Could you check a few things on this model? Use its own coordinates, in mm. Round coordinates to 2 decimals unless told otherwise and drop trailing zeros. Order: outer loops, then holes, each group sorted by start corner. A loop starts at its lowest first (then second) coordinate and runs counter-clockwise, first axis right, second up. Notation, with made-up numbers: M 3.5,-28.75 L 23.5,-28.75 A22 ccw 23.5,10.25 Z; hole C 43,-22 d6. An arc over 180 degrees is marked long. Write each question's results on one line, items separated by ' | '. Start each with the question number.
1. Please list where these lines run through material, in increasing order: L1, parallel to Y at x = -115.5, z = -0.55; L2, parallel to Y at x = -35.5, z = 0.65; L3, parallel to X at y = -23, z = 0.8.
2. I'm going to push flat-ended pins straight in: pin 1 (0.8 mm diameter, centred on x = -42, z = -0.5, fed in from +Y); pin 2 (1 mm diameter, centred on x = -39.5, z = -1, fed in from -Y); pin 3 (1.1 mm diameter, centred on x = -37, z = 0.5, fed in from +Y). Where does each tip first touch, or does it pass through?
3. Suppose I cut it at A-A on z = 0.4. Write out the boundary of the cut face in (x, y).
4. Suppose I cut it at B-B on y = -19. Write out the boundary of the cut face in (x, z).
5. Suppose I cut it at C-C on x = -108.5. Write out the boundary of the cut face in (y, z), and give its area (3 significant figures).
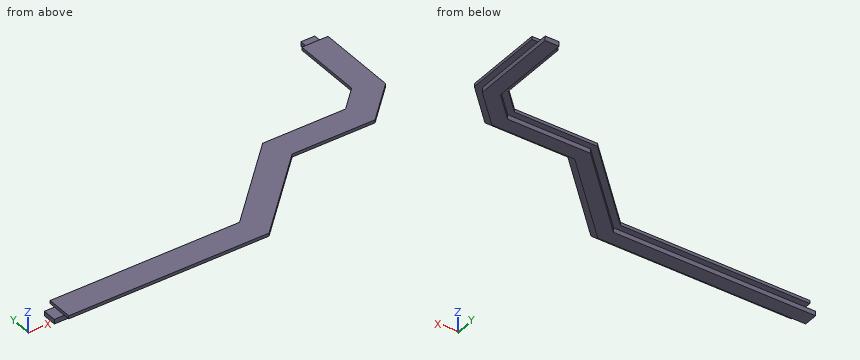
Autodesk Inventor part; units mm, degrees
ref_plane "YZ Plane" through (0, 0, 0) normal (1, 0, 0) x (0, 1, 0)
ref_plane "XZ Plane" through (0, 0, 0) normal (0, 1, 0) x (-1, 0, 0)
ref_plane "XY Plane" through (0, 0, 0) normal (0, 0, 1) x (1, 0, 0)
sketch "Эскиз1" plane through (0, 0, 0) normal (0, 0, 1) x (1, 0, 0)
  line L0 (-75.0711, -58) -> (-141.1512, -58)
  line L1 (-141.1512, -58) -> (-141.1512, -4.9289)
  line L2 (-141.1512, -4.9289) -> (-133.2223, 3)
  line L3 (-14, 3) -> (-133.2223, 3)
  line L4 (-14, 3) -> (-14, -24.0711)
  line L5 (-14, -24.0711) -> (-21.9289, -32)
  line L6 (-21.9289, -32) -> (-49.0711, -32)
  line L7 (-49.0711, -32) -> (-75.0711, -58)
  line L8 (-131.1512, -2) -> (-136.1512, -7)
  line L9 (-136.1512, -7) -> (-136.1512, -13.8712)
  line L10 (-136.1512, -13.8712) -> (-136.1512, -19.5281)
  line L11 (-136.1512, -19.5281) -> (-136.1512, -26.3992)
  line L12 (-136.1512, -26.3992) -> (-136.1512, -27)
  line L13 (-136.1512, -27) -> (-131.0951, -27)
  line L14 (-131.0951, -27) -> (-124.224, -27)
  line L15 (-124.224, -27) -> (-118.5671, -27)
  line L16 (-118.5671, -27) -> (-111.696, -27)
  line L17 (-111.696, -27) -> (-106.0391, -27)
  line L18 (-106.0391, -27) -> (-99.168, -27)
  line L19 (-99.168, -27) -> (-93.5111, -27)
  line L20 (-93.5111, -27) -> (-86.64, -27)
  line L21 (-86.64, -27) -> (-80.9831, -27)
  line L22 (-80.9831, -27) -> (-74.112, -27)
  line L23 (-74.112, -27) -> (-68.4551, -27)
  line L24 (-68.4551, -27) -> (-61.584, -27)
  line L25 (-61.584, -27) -> (-55.9271, -27)
  line L26 (-55.9271, -27) -> (-49.056, -27)
  line L27 (-49.056, -27) -> (-43.3991, -27)
  line L28 (-43.3991, -27) -> (-36.528, -27)
  line L29 (-36.528, -27) -> (-30.8711, -27)
  line L30 (-30.8711, -27) -> (-24, -27)
  line L31 (-24, -27) -> (-19, -22)
  line L32 (-19, -22) -> (-19, -15.1289)
  line L33 (-19, -15.1289) -> (-19, -9.472)
  line L34 (-19, -9.472) -> (-19, -2.6009)
  line L35 (-19, -2.6009) -> (-19, -2)
  line L36 (-19, -2) -> (-24.056, -2)
  line L37 (-24.056, -2) -> (-30.9271, -2)
  line L38 (-30.9271, -2) -> (-36.584, -2)
  line L39 (-36.584, -2) -> (-43.4551, -2)
  line L40 (-43.4551, -2) -> (-49.112, -2)
  line L41 (-49.112, -2) -> (-55.9831, -2)
  line L42 (-55.9831, -2) -> (-61.64, -2)
  line L43 (-61.64, -2) -> (-68.5111, -2)
  line L44 (-68.5111, -2) -> (-74.168, -2)
  line L45 (-74.168, -2) -> (-81.0391, -2)
  line L46 (-81.0391, -2) -> (-86.696, -2)
  line L47 (-86.696, -2) -> (-93.5671, -2)
  line L48 (-93.5671, -2) -> (-99.224, -2)
  line L49 (-99.224, -2) -> (-106.0951, -2)
  line L50 (-106.0951, -2) -> (-111.752, -2)
  line L51 (-111.752, -2) -> (-118.6231, -2)
  line L52 (-118.6231, -2) -> (-124.28, -2)
  line L53 (-124.28, -2) -> (-131.1512, -2)
  line L54 (-141.1512, -69.9) -> (-42.8584, -69.9)
  line L55 (-141.1512, -63) -> (-141.1512, -69.9)
  line L56 (-141.1512, -63) -> (-73, -63)
  line L57 (-73, -63) -> (-47, -37)
  line L58 (-47, -37) -> (-19.8579, -37)
  line L59 (-19.8579, -37) -> (-9, -26.1421)
  line L60 (-9, -26.1421) -> (-9, 3)
  line L61 (-9, 3) -> (-2, 3)
  line L62 (-2, -29.0416) -> (-2, 3)
  line L63 (-42.8584, -69.9) -> (-2, -29.0416)
  line L64 (-73.0828, -62.8) -> (-141.3512, -62.8)
  line L65 (-141.3512, -62.8) -> (-141.3512, -70.1)
  line L66 (-141.3512, -70.1) -> (-42.7755, -70.1)
  line L67 (-42.7755, -70.1) -> (-1.8, -29.1245)
  line L68 (-1.8, -29.1245) -> (-1.8, 3.2)
  line L69 (-1.8, 3.2) -> (-9.2, 3.2)
  line L70 (-9.2, 3.2) -> (-9.2, -26.0593)
  line L71 (-9.2, -26.0593) -> (-19.9407, -36.8)
  line L72 (-19.9407, -36.8) -> (-47.0828, -36.8)
  line L73 (-47.0828, -36.8) -> (-73.0828, -62.8)
  line L74 (-141.3512, -58.2) -> (-74.9882, -58.2)
  line L75 (-74.9882, -58.2) -> (-48.9882, -32.2)
  line L76 (-48.9882, -32.2) -> (-21.8461, -32.2)
  line L77 (-21.8461, -32.2) -> (-13.8, -24.1539)
  line L78 (-13.8, -24.1539) -> (-13.8, 3.2)
  line L79 (-13.8, 3.2) -> (-133.3051, 3.2)
  line L80 (-133.3051, 3.2) -> (-141.3512, -4.8461)
  line L81 (-141.3512, -4.8461) -> (-141.3512, -58.2)
  line L82 (-141.1512, -58) -> (-141.1512, -66.7)
  line L83 (-5.3, 3) -> (-14, 3)
  line L84 (-44.9289, -42) -> (-65.9289, -63)
  line L85 (-65.9289, -63) -> (-45.8579, -63)
  line L86 (-45.8579, -63) -> (-24.8579, -42)
  line L87 (-24.8579, -42) -> (-44.9289, -42)
  point P0 (-9.2, 3)
  point P1 (-13.8, 3)
  point P2 (-141.1512, -58.2)
  point P3 (-141.1512, -62.8)
  dimension "d10" = 0.2
  dimension "d11" = 0.2
extrude "Выдавливание1" add sketch "Эскиз1" against normal blind 1.5 contours L74 L75 L76 L77 L78 L83 L70 L71 L72 L73 L64 L82
sketch "Эскиз2" plane through (0, 0, 0) normal (0, 0, 1) x (1, 0, 0)
  line L0 (-19.9407, -36.8) -> (-47.0828, -36.8)
  line L1 (-47.0828, -36.8) -> (-73.0828, -62.8)
  line L2 (-73.0828, -62.8) -> (-141.1512, -62.8)
  line L3 (-141.1512, -62.8) -> (-141.1512, -58.2)
  line L4 (-141.1512, -58.2) -> (-74.9882, -58.2)
  line L5 (-74.9882, -58.2) -> (-48.9882, -32.2)
  line L6 (-48.9882, -32.2) -> (-21.8461, -32.2)
  line L7 (-21.8461, -32.2) -> (-13.8, -24.1539)
  line L8 (-13.8, -24.1539) -> (-13.8, 3)
  line L9 (-13.8, 3) -> (-9.2, 3)
  line L10 (-9.2, 3) -> (-9.2, -26.0593)
  line L11 (-9.2, -26.0593) -> (-19.9407, -36.8)
  line L12 (-75.8167, -56.2) -> (-143.1512, -56.2)
  line L13 (-143.1512, -56.2) -> (-143.1512, -64.8)
  line L14 (-143.1512, -64.8) -> (-72.2544, -64.8)
  line L15 (-72.2544, -64.8) -> (-46.2544, -38.8)
  line L16 (-46.2544, -38.8) -> (-19.1123, -38.8)
  line L17 (-19.1123, -38.8) -> (-7.2, -26.8877)
  line L18 (-7.2, -26.8877) -> (-7.2, 5)
  line L19 (-7.2, 5) -> (-15.8, 5)
  line L20 (-15.8, 5) -> (-15.8, -23.3255)
  line L21 (-15.8, -23.3255) -> (-22.6745, -30.2)
  line L22 (-22.6745, -30.2) -> (-49.8167, -30.2)
  line L23 (-49.8167, -30.2) -> (-75.8167, -56.2)
  line L24 (-138.1512, -66.9) -> (-138.1512, -63)
  line L25 (-14, 0) -> (-5.3, 0)
  line L26 (-7.2, 0) -> (-7.2, -0.3)
  line L27 (-7.2, -0.3) -> (-15.8, -0.3)
  line L28 (-138.1512, -64.8) -> (-137.8512, -64.8)
  line L29 (-137.8512, -64.8) -> (-137.8512, -56.2)
  dimension "d12" = 2
  dimension "d13" = 0.3
  dimension "d14" = 0.3
extrude "Выдавливание2" add sketch "Эскиз2" along normal blind 1 contours L11 L10 L27 L18 L17 L16 L15 L14 L29 L2 L1 L0 | L0 L1 L2 L29 L4 L5 L6 L7 L8 L27 L10 L11 | L8 L7 L6 L5 L4 L29 L12 L23 L22 L21 L20 L27
properties part number "right_line"
Filled sheet:
1) L1: y = -62.8 to -58.2 | L2: y = -38.8 to -30.2 | L3: x = -15.8 to -7.2
2) pin 1: stops at y = -32.2 | pin 2: stops at y = -36.8 | pin 3: stops at y = -30.2
3) outline: M -137.85,-64.8 L -72.25,-64.8 L -46.25,-38.8 L -19.11,-38.8 L -7.2,-26.89 L -7.2,-0.3 L -15.8,-0.3 L -15.8,-23.33 L -22.67,-30.2 L -49.82,-30.2 L -75.82,-56.2 L -137.85,-56.2 Z
4) outline: M -15.8,0 L -13.8,0 L -13.8,-1.5 L -9.2,-1.5 L -9.2,0 L -7.2,0 L -7.2,1 L -15.8,1 Z
5) outline: M -64.8,0 L -62.8,0 L -62.8,-1.5 L -58.2,-1.5 L -58.2,0 L -56.2,0 L -56.2,1 L -64.8,1 Z | area: 15.5 mm^2
